```python
from build123d import *

# Parameters (mm, degrees)
SKETCH1_R                = 8.8
SKETCH1_R_2              = 7.6
BOSS_EXTRUDE1_DEPTH      = 10
SKETCH2_W                = 18.171732103
SKETCH2_H                = 2
CUT_EXTRUDE1_DEPTH       = 8
SKETCH3_R                = 8.8
BOSS_EXTRUDE2_DEPTH      = 1
SKETCH4_R                = 1.75
CUT_EXTRUDE2_DEPTH       = 17.609635758
FILLET1_R                = 0.5
FILLET3_R                = 1.5
CIRPATTERN1_COUNT        = 2
FILLET1_OF_CIRPATTERN1_R = 0.5
FILLET3_OF_CIRPATTERN1_R = 1.5
SKETCH5_R                = 2.95
SKETCH5_R_2              = 1.75
BOSS_EXTRUDE3_DEPTH      = 3
FILLET6_R                = 1


with BuildPart() as part:
    # Sketch1 → Boss-Extrude1 (new body)
    with BuildSketch(Plane(origin=(0, 0, 0), x_dir=(1, 0, 0), z_dir=(0, 1, 0))):
        with Locations(Location((0, 0, 0), (0, 0, 270))):
            Circle(SKETCH1_R)
        with Locations(Location((0, 0, 0), (0, 0, 270))):
            Circle(SKETCH1_R_2, mode=Mode.SUBTRACT)
    extrude(amount=BOSS_EXTRUDE1_DEPTH)

    # Sketch2 → Cut-Extrude1 (cut)
    with BuildSketch(Plane.XZ):
        with Locations((9.085866052, 0)):
            Rectangle(SKETCH2_W, SKETCH2_H)
    cut_extrude1 = extrude(amount=-CUT_EXTRUDE1_DEPTH, mode=Mode.SUBTRACT)

    # Sketch3 → Boss-Extrude2 (add)
    with BuildSketch(Plane(origin=(0, 10, 0), x_dir=(1, 0, 0), z_dir=(0, 1, 0))):
        with Locations(Location((0, 0, 0), (0, 0, 6.524978844))):
            Circle(SKETCH3_R)
    extrude(amount=BOSS_EXTRUDE2_DEPTH)

    # Sketch4 → Cut-Extrude2 (cut, through all)
    with BuildSketch(Plane(origin=(0, 11, 0), x_dir=(1, 0, 0), z_dir=(0, 1, 0))):
        with Locations(Location((0, 0, 0), (0, 0, 270))):
            Circle(SKETCH4_R)
    extrude(amount=-CUT_EXTRUDE2_DEPTH, mode=Mode.SUBTRACT)

    # Fillet1
    fillet1_edges = [part.edges().sort_by_distance(p)[0] for p in [
        (8.138460239, 8, -1),
        (8.138460239, 8, 1),
    ]]
    fillet(fillet1_edges, radius=FILLET1_R)

    # Fillet3
    fillet3_edges = [part.edges().sort_by_distance(p)[0] for p in [
        (8.138460239, 0, 1),
        (8.138460239, 0, -1),
    ]]
    fillet(fillet3_edges, radius=FILLET3_R)

    # CirPattern1: Cut-Extrude1 ×2 about axis
    cirpattern1_axis = Axis((0, 0, 0), (0, -1, 0))
    for i in range(1, CIRPATTERN1_COUNT):
        add(cut_extrude1.rotate(cirpattern1_axis, i * 360 / CIRPATTERN1_COUNT), mode=Mode.SUBTRACT)

    # Fillet1 of CirPattern1
    fillet1_of_cirpattern1_edges = [part.edges().sort_by_distance(p)[0] for p in [
        (-8.138460239, 8, 1),
        (-8.138460239, 8, -1),
    ]]
    fillet(fillet1_of_cirpattern1_edges, radius=FILLET1_OF_CIRPATTERN1_R)

    # Fillet3 of CirPattern1
    fillet3_of_cirpattern1_edges = [part.edges().sort_by_distance(p)[0] for p in [
        (-8.138460239, 0, -1),
        (-8.138460239, 0, 1),
    ]]
    fillet(fillet3_of_cirpattern1_edges, radius=FILLET3_OF_CIRPATTERN1_R)

    # Sketch5 → Boss-Extrude3 (add)
    with BuildSketch(Plane.XZ.offset(-10)):
        with Locations(Location((0, 0, 0), (0, 0, 90))):
            Circle(SKETCH5_R)
        with Locations(Location((0, 0, 0), (0, 0, 90))):
            Circle(SKETCH5_R_2, mode=Mode.SUBTRACT)
    extrude(amount=BOSS_EXTRUDE3_DEPTH)

    # Fillet6
    fillet6_edges = [part.edges().sort_by_distance(p)[0] for p in [
        (0, 10, -7.6),
    ]]
    fillet(fillet6_edges, radius=FILLET6_R)


solid = part.part
```
Could you check a few things on this model? Use its own coordinates, in mm. A direction names the side the tool comes from. Coordinates: 2 decimals unless noted, no trailing zeros. Write each loop counter-clockwise with the first axis right and the second up, starting at its lowest first coordinate (ties: lowest second). Pieces come first, ordered by that corner, then holes. Notation, with made-up numbers: (48, 87) -> (102, 87) arc R4 cw to (102, 92) -> close; hole circle Ø3 at (61.25, 37). An arc over 180 degrees is marked (long way). One line per question, with ' | ' between items. Start each with the question number.
1. If we section it at A-A (y = 5.75): Please give me the cut outline in (x, z), and give its area (3 significant figures).
2. For faces 4 (the face through (-8, 8, 0)), 5 (the face through (7.97, 0.43, 1.45)), 6 (the face through (-7.42, 4.44, -1.65)), which set-ups out of +Z, -Z, +X, -X, +Y, -Y let a thin tool reach every point of the face, with its end or its side?
3. If we section it at C-C (y = 10.75): Please give me the cut outline in (x, z), and give its area (3 significant figures).
4. Will these pins go through, and if not, where does the flat tip stop? P1, Ø4, axis at x = -2.5, y = 8, coming from the +Z side; P2, Ø2, axis at y = 4.5, z = -3.5, coming from the -X side; P3, Ø0.5, axis at x = -8, z = 0, coming from the -Y side.
5. Please list where these lines run through material, in increasing order: line 1 along X through (y, z) = (8.1, 0); line 2 along Z through (x, y) = (-1.25, 9.75); line 3 along Y through (x, z) = (-5.25, 1.5).
6. Thinking about a two-plate mould opening in X: for faces 1 (the face through (-8, 4, 1)), 2 (the face through (8.157, 5.423, 3.301)), 3 (the face through (2, 7, 0)), which applies, pulls with the +X half, pulls with the -X half, needs draft (parallel to the pull), parting line crosses it, or undercut?
Return value:
1) outline: (-8.74, -1) arc R8.8 ccw to (8.74, -1) -> (7.53, -1) arc R7.6 cw to (-7.53, -1) -> close; (-8.74, 1) -> (-7.53, 1) arc R7.6 cw to (7.53, 1) -> (8.74, 1) arc R8.8 ccw to start | area: 57.0 mm²
2) face 4: -X, -Y | face 5: +X, -X, -Y | face 6: -Y
3) outline: circle Ø17.6 at (0, 0); hole circle Ø3.5 at (0, 0) | area: 234 mm²
4) P1: stops at z = 8.79 | P2: stops at x = -8.44 | P3: stops at y = 8
5) line 1: x = -8.8 to -7.6, -2.95 to -1.75, 1.75 to 2.95, 7.6 to 8.8 | line 2: z = -8.71 to -7.15, -2.67 to -1.22, 1.22 to 2.67, 7.15 to 8.71 | line 3: y = 10 to 11
6) face 1: needs draft | face 2: parting line crosses it | face 3: undercut
